```python
from build123d import *

# Parameters (mm, degrees)
BOSS_EXTRUDE1_DEPTH = 80
BOSS_EXTRUDE2_DEPTH = 7.16
SKETCH3_R           = 6
CUT_EXTRUDE1_DEPTH  = 7.16
CUT_EXTRUDE6_DEPTH  = 95
CUT_EXTRUDE7_DEPTH  = 85
CHAMFER3_SIZE       = 7
CHAMFER3_SIZE2      = 12.628334287
SCALE1_SCALE        = 0.714781685
SCALE2_SCALE        = 0.5
SCALE3_SCALE        = 1.5


with BuildPart() as part:
    # Sketch1 → Boss-Extrude1 (new body)
    with BuildSketch(Plane(origin=(0, 0, 0), x_dir=(0, 0, -1), z_dir=(1, 0, 0))):
        with BuildLine():
            Line((-43.05875576, 0), (51.94124424, 0))
            ThreePointArc((51.94124424, 0), (73.154447675, 8.786796564), (81.94124424, 30))
            Line((81.94124424, 30), (81.94124424, 155))
            Line((81.94124424, 155), (74.78124424, 155))
            Line((74.78124424, 155), (74.78124424, 30))
            ThreePointArc((74.78124424, 30), (68.091563122, 13.849681118), (51.94124424, 7.16))
            Line((51.94124424, 7.16), (-43.05875576, 7.16))
            Line((-43.05875576, 7.16), (-43.05875576, 0))
        make_face()
    extrude(amount=BOSS_EXTRUDE1_DEPTH)

    # Sketch2 → Boss-Extrude2 (add)
    with BuildSketch(Plane.XY.offset(-74.78124424)):
        Polygon((0, 155), (68.44375, 188.037147061), (80, 155), align=None)
    extrude(amount=-BOSS_EXTRUDE2_DEPTH)

    # Sketch3 → Cut-Extrude1 (cut)
    with BuildSketch(Plane.XY.offset(-74.78124424)):
        with Locations((63.851173507, 176.937147061)):
            Circle(SKETCH3_R)
        with Locations((8, 149.978316888)):
            Circle(SKETCH3_R)
    extrude(amount=-CUT_EXTRUDE1_DEPTH, mode=Mode.SUBTRACT)

    # Sketch6 → Cut-Extrude6 (cut)
    with BuildSketch(Plane.XY.offset(43.05875576)):
        Polygon((80, 0), (64.645330449, 7.16), (80, 7.16), align=None)
    extrude(amount=-CUT_EXTRUDE6_DEPTH, mode=Mode.SUBTRACT)

    # Sketch10 → Cut-Extrude7 (cut)
    with BuildSketch(Plane(origin=(0, 115, 0), x_dir=(-1, 0, 0), z_dir=(0, -1, 0))):
        Polygon((-80, 81.94124424), (-60, 74.78124424), (-80, 74.78124424), align=None)
    extrude(amount=CUT_EXTRUDE7_DEPTH, mode=Mode.SUBTRACT)

    # Chamfer3
    chamfer3_edges = [part.edges().sort_by_distance(p)[0] for p in [
        (80, 13.849681118, -68.091563122),
    ]]
    chamfer3_side = [part.faces().sort_by_distance(p)[0] for p in [
        (80, 13.077563731, -68.863680509),
    ]]
    chamfer(chamfer3_edges, length=CHAMFER3_SIZE, length2=CHAMFER3_SIZE2, reference=chamfer3_side[0])


with BuildPart() as part_1:
    # Scale1: scaled about (37.569148968, 54.949559207, -51.822054035)
    add(part.part.scale(SCALE1_SCALE).moved(Location((10.715409355, 15.672620673, -14.780598919))))


with BuildPart() as part_2:
    # Scale2: scaled about (37.569148968, 54.949559207, -51.822054035)
    add(part_1.part.scale(SCALE2_SCALE).moved(Location((18.784574484, 27.474779604, -25.911027018))))


with BuildPart() as part_3:
    # Scale3: scaled about (37.569148968, 54.949559207, -51.822054035)
    add(part_2.part.scale(SCALE3_SCALE).moved(Location((-18.784574484, -27.474779604, 25.911027018))))


solid = part_3.part
```
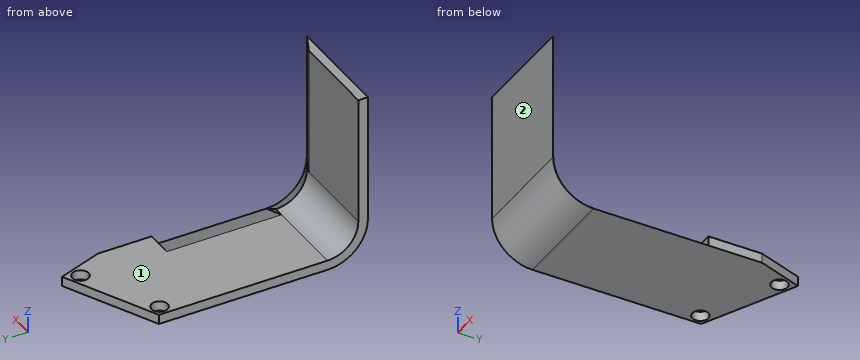
CAD build for the part. Positions are in the model's coordinates, mm. Face numbers are marked on the shaded views. A direction names the side the tool comes from. Coordinates: 2 decimals unless noted, no trailing zeros. Order: outer loops, then holes, each group sorted by start corner. A loop starts at its lowest first (then second) coordinate and runs counter-clockwise, first axis right, second up. Notation, with made-up numbers: (-11.5, 44.25) - (8.5, 44.25) arc R32 cw to (8.5, 73.25) - close; hole circle Ø4 at (40, 40.25). An arc over 180 degrees is marked (long way). Answer in a Markdown table with one row per item.
1. Flat gauge pins, fed straight in: P1, Ø6, axis at x = 38.5, y = 116, coming from the +Z side; P2, Ø5, axis at x = 51.66, y = 120.35, coming from the -Z side; P3, Ø4, axis at x = 54, z = -66, coming from the -Y side; P4, Ø10.5, axis at x = 33, z = -31, coming from the +Y side. Where does each tip first touch, or does it go through?
Answer:
| item | result |
|---|---|
| P1 | z = -64.13 |
| P2 | through |
| P3 | y = 31 |
| P4 | y = 29.33 |
2. Slice it at C-C, the plane x = 28.5. List the corners of the cut face in (y, z), then the cut area to 3 significant figures.
Answer:
| item | result |
|---|---|
| outline | (25.49, -51.89) arc R16.08 ccw to (41.57, -67.97) - (113.93, -67.97) - (113.93, -64.13) - (41.57, -64.13) arc R12.24 cw to (29.33, -51.89) - (29.33, -0.96) - (25.49, -0.96) - close |
| area | 559 mm² |
3. Slice it at B-B, the plane z = -24. List the corners of the cut face in (x, y).
Answer:
| item | result |
|---|---|
| outline | (17.43, 25.49) - (60.32, 25.49) - (52.08, 29.33) - (17.43, 29.33) - close |
4. Drill centre lines: L1, parallel to Y at x = 43, z = -14; L2, parallel to Z at x = 20.5, y = 84; L3, parallel to X at y = 38, z = -65. Where is each one in solid material? Low to high. Write a range as from..to.
Answer:
| item | result |
|---|---|
| L1 | 25.49..29.33 |
| L2 | -67.97..-64.13 |
| L3 | 17.43..55.98 |
5. Slice it at D-D, the plane y = 47. List the corners of the cut face in (x, z), then the cut area to 3 significant figures.
Answer:
| item | result |
|---|---|
| outline | (17.43, -67.97) - (60.32, -67.97) - (49.59, -64.13) - (17.43, -64.13) - close |
| area | 144 mm² |
6. Slice it at A-A, the plane x = 20. List the corners of the cut face in (y, z).
Answer:
| item | result |
|---|---|
| outline | (25.49, -51.89) arc R16.08 ccw to (41.57, -67.97) - (103.17, -67.97) - (103.17, -64.13) - (41.57, -64.13) arc R12.24 cw to (29.33, -51.89) - (29.33, -0.96) - (25.49, -0.96) - close; (108.61, -67.97) - (109.83, -67.97) - (109.83, -64.13) - (108.61, -64.13) - close |
7. 3-axis set-ups, long thin cutter, end or side, ignore diameter. For the marked faces 1 and 2: which of +Z, -Z, +X, -X, +Y, -Y reach the whole face in a straight line?
Answer:
| item | result |
|---|---|
| face 1 | +Z, +X, -X, +Y |
| face 2 | +Z, -Z, +X, -X, -Y |
